Geometry: final body of the model. Coordinates: model frame, mm. A direction names the side the tool comes from. Round coordinates to 2 decimals unless told otherwise and drop trailing zeros. Order: outer loops, then holes, each group sorted by start corner. A loop starts at its lowest first (then second) coordinate and runs counter-clockwise, first axis right, second up. Notation, with made-up numbers: (37.25, 58) - (76.25, 58) arc R14 ccw to (76.25, 70) - close; hole circle Ø9 at (67.5, -23.5). An arc over 180 degrees is marked (long way). Put each result on its own line as item: value. Start each with the question number.
(1) Access query for faces 1 (the face through (-76.518, 0, 2)), 2 (the face through (-87.63, -2, -3)), 3 (the face through (-73.342, 0, 2)). Directions: +Z, -Z, +X, -X, +Y, -Y. A direction counts if a zero-diameter tool reaches every point of the face in a straight line with its end or side. Return the directions, or none.
(2) Section A-A (y = 43.5). Output: boundary loops of the cut face in (x, z).
(3) Section B-B (x = -31.5). Output: boundary loops of the cut face in (y, z) (3 decimals).
(4) Material intervals for L1, parallel to Y at x = 81.28, z = -3.8 (1 decimal); L2, parallel to Z at x = -80, y = 18.5, sorted ascending. Write a range as [from, to].
(5) Pin query (flat end, axial travel): P1, Ø4, axis at x = 81.28, y = -94.615, coming from the +Z side; P2, Ø2.5, axis at x = 81.28, y = 94.615, coming from the -Z side; P3, Ø2.5, axis at x = -74.5, z = 3, coming from the -Y side; P4, Ø3.5, axis at x = -75.5, z = 3.5, coming from the +Y side. Return the tip coordinate at first contact, or that it passes through.
from build123d import *

# Parameters (mm, degrees)
SKETCH1_W           = 175.26
SKETCH1_H           = 240.03
BOSS_EXTRUDE1_DEPTH = 5.08
SKETCH2_R           = 1.5875
CUT_EXTRUDE1_DEPTH  = 149.689016155
SKETCH3_W           = 3.175
SKETCH3_H           = 25.4
BOSS_EXTRUDE2_DEPTH = 12.7
SKETCH4_W           = 7.62
SKETCH4_H           = 20.32
CUT_EXTRUDE2_DEPTH  = 202.189055322
FILLET1_R           = 2.54


with BuildPart() as part:
    # Sketch1 → Boss-Extrude1 (new body)
    with BuildSketch(Plane.XY):
        Rectangle(SKETCH1_W, SKETCH1_H)
    extrude(amount=-BOSS_EXTRUDE1_DEPTH)

    # Sketch2 → Cut-Extrude1 (cut, through all)
    with BuildSketch(Plane.XY):
        with Locations((81.28, 100.965)):
            Circle(SKETCH2_R)
        with Locations((81.28, 94.615)):
            Circle(SKETCH2_R)
        with Locations(Location((81.28, -94.615, 0), (0, 0, 180))):
            Circle(SKETCH2_R)
        with Locations(Location((81.28, -100.965, 0), (0, 0, 180))):
            Circle(SKETCH2_R)
    extrude(amount=-CUT_EXTRUDE1_DEPTH, mode=Mode.SUBTRACT)

    # Sketch3 → Boss-Extrude2 (add)
    with BuildSketch(Plane.XY):
        with Locations((-74.93, 0)):
            Rectangle(SKETCH3_W, SKETCH3_H)
    extrude(amount=BOSS_EXTRUDE2_DEPTH)

    # Sketch4 → Cut-Extrude2 (cut, through all)
    with BuildSketch(Plane(origin=(-73.3425, 0, 0), x_dir=(0, 0, -1), z_dir=(1, 0, 0))):
        with Locations((-6.35, 0)):
            Rectangle(SKETCH4_W, SKETCH4_H)
    extrude(amount=-CUT_EXTRUDE2_DEPTH, mode=Mode.SUBTRACT)

    # Fillet1
    fillet1_edges = [part.edges().sort_by_distance(p)[0] for p in [
        (-74.93, 12.7, 12.7),
        (-74.93, -12.7, 12.7),
        (-74.93, 10.16, 2.54),
        (-74.93, -10.16, 2.54),
        (-74.93, -10.16, 10.16),
        (-74.93, 10.16, 10.16),
    ]]
    fillet(fillet1_edges, radius=FILLET1_R)


solid = part.part
Checks:
1. face 1: +Z, -X, +Y, -Y
1. face 2: +Z, -Z, -X, +Y, -Y
1. face 3: +Z, +X, +Y, -Y
2. outline: (-87.63, -5.08) - (87.63, -5.08) - (87.63, 0) - (-87.63, 0) - close
3. outline: (-120.015, -5.08) - (120.015, -5.08) - (120.015, 0) - (-120.015, 0) - close
4. L1: y = [-120, -102.6], [-99.4, -96.2], [-93, 93], [96.2, 99.4], [102.6, 120]
4. L2: z = [-5.08, 0]
5. P1: stops at z = 0
5. P2: passes through
5. P3: stops at y = -12.7
5. P4: stops at y = 12.7
